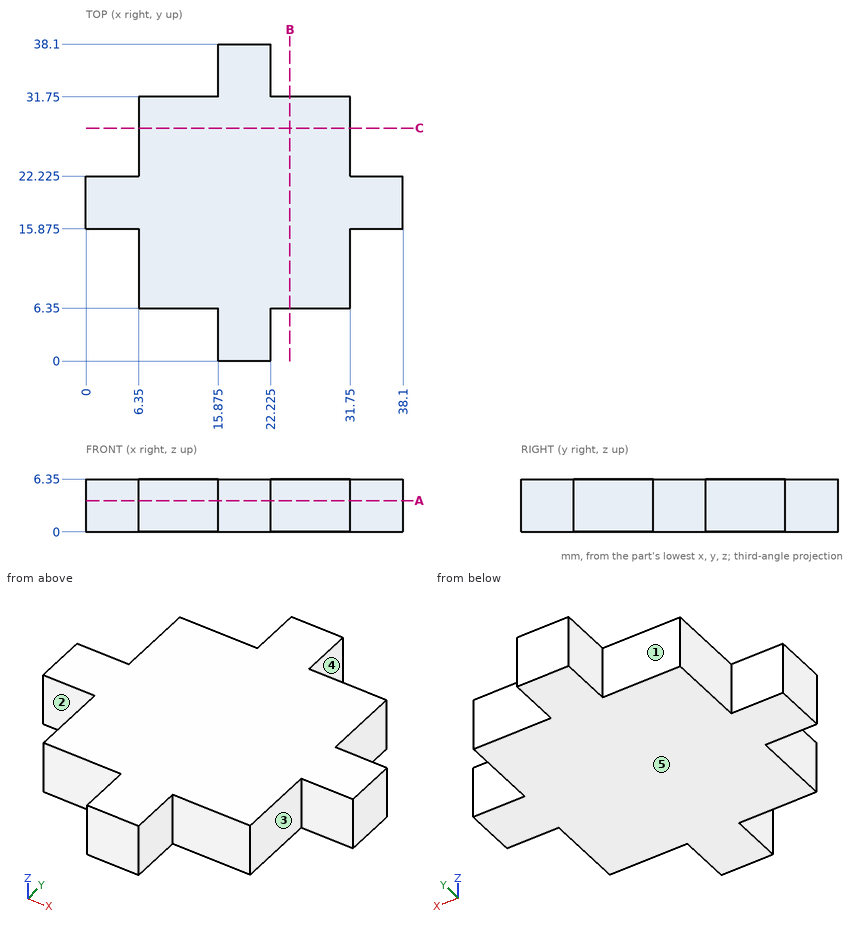
Print and shaded views of the part. All mm, measured from the part's lowest x, y and z. A direction names the side the tool comes from. Give positions to 0.01 mm unless a question says otherwise; leave off trailing zeros. Order: outer loops, then holes, each group sorted by start corner. A loop starts at its lowest first (then second) coordinate and runs counter-clockwise, first axis right, second up. Notation, with made-up numbers: (48, 53) - (103, 53) arc R5 cw to (103, 62) - close; hole circle Ø6 at (60, 28). An arc over 180 degrees is marked (long way). One line per item, written item: value.
Item 1: Wall check: line 1 (X direction, y = 14, z = 3.5); line 2 (Y direction, x = 34.5, z = 1.5) (3 decimals). Give the ranges that are in metal, low to high.
Response values:
line 1: 6.35 to 31.75
line 2: 15.875 to 22.225
Item 2: Pin check, flat tips, straight feed: pin 1 Ø1.9 at (x, z) = (9.5, 4) entering from -Y; pin 2 Ø1.9 at (x, z) = (2.5, 3.5) entering from -Y (3 decimals); pin 3 Ø3 at (y, z) = (33.5, 3) entering from +X (3 decimals). Stop position of each tip, or through.
Response values:
pin 1: y = 6.35
pin 2: y = 15.875
pin 3: x = 22.225
Item 3: Slice it at A-A (z = 3.75). List the corners of the cut face in (x, y) (3 decimals).
Response values:
outline: (0, 15.875) - (6.35, 15.875) - (6.35, 6.35) - (15.875, 6.35) - (15.875, 0) - (22.225, 0) - (22.225, 6.35) - (31.75, 6.35) - (31.75, 15.875) - (38.1, 15.875) - (38.1, 22.225) - (31.75, 22.225) - (31.75, 31.75) - (22.225, 31.75) - (22.225, 38.1) - (15.875, 38.1) - (15.875, 31.75) - (6.35, 31.75) - (6.35, 22.225) - (0, 22.225) - close
Item 4: Slice it at B-B (x = 24.5). List the corners of the cut face in (y, z), then the cut area to 3 significant figures.
Response values:
outline: (6.35, 0) - (31.75, 0) - (31.75, 6.35) - (6.35, 6.35) - close
area: 161 mm2
Item 5: Tool access for the marked faces 1, 2, 3, 4 and 5: list every direction of +Z, -Z, +X, -X, +Y, -Y with a clear straight run to the whole face (end or side of a thin tool).
Response values:
face 1: +Z, -Z, -X, +Y
face 2: +Z, -Z, -X, -Y
face 3: +Z, -Z, +X, -Y
face 4: +Z, -Z, +X, +Y
face 5: -Z, +X, -X, +Y, -Y
